Autodesk Inventor part; units mm, degrees
ref_plane "YZ Plane" through (0, 0, 0) normal (1, 0, 0) x (0, 1, 0)
ref_plane "XZ Plane" through (0, 0, 0) normal (0, 1, 0) x (-1, 0, 0)
ref_plane "XY Plane" through (0, 0, 0) normal (0, 0, 1) x (1, 0, 0)
sketch "Sketch1" plane through (0, 0, 0) normal (0, 0, 1) x (1, 0, 0)
  line L0 (15.75, -68) -> (15.75, -43)
  line L1 (15.75, -43) -> (18.75, -43)
  line L2 (18.75, -43) -> (18.75, -68)
  line L3 (43.75, -58) -> (43.75, 0)
  arc A0 (33.75, -68) -> (43.75, -58) centre (33.75, -58) ccw
  circle A1 centre (33.75, -58) radius 5
  line L4 (13.75, 0) -> (13.75, 3)
  line L5 (13.75, 3) -> (3.75, 3)
  line L6 (3.75, 3) -> (3.75, 0)
  line L7 (28.75, 0) -> (28.75, 3)
  line L8 (28.75, 3) -> (38.75, 3)
  line L9 (38.75, 3) -> (38.75, 0)
  line L10 (43.75, 0) -> (38.75, 0)
  line L11 (28.75, 0) -> (13.75, 0)
  line L12 (3.75, 0) -> (0, 0)
  line L13 (0, 0) -> (0, -21.8755)
  line L14 (5.75, -68) -> (0.0154, -22.1236)
  arc A2 (0, -21.8755) -> (0.0154, -22.1236) centre (2, -21.8755) ccw
  line L15 (33.75, -68) -> (18.75, -68)
  line L16 (15.75, -68) -> (5.75, -68)
  line L17 (26.8402, -47) -> (33.75, -47)
  line L18 (38.75, -42) -> (38.75, -10)
  line L19 (22.368, -44.2361) -> (19.2779, -38.0557)
  line L20 (33.75, -5) -> (23.75, -5)
  line L21 (18.75, -10) -> (18.75, -35.8197)
  arc A3 (23.75, -5) -> (18.75, -10) centre (23.75, -10) ccw
  arc A4 (38.75, -10) -> (33.75, -5) centre (33.75, -10) ccw
  arc A5 (33.75, -47) -> (38.75, -42) centre (33.75, -42) ccw
  arc A6 (22.368, -44.2361) -> (26.8402, -47) centre (26.8402, -42) ccw
  arc A7 (18.75, -35.8197) -> (19.2779, -38.0557) centre (23.75, -35.8197) ccw
  point P0 (43.75, -69.5)
  point P1 (0, -22)
  point P2 (23.75, -47)
  point P3 (18.75, -37)
  dimension "d7" = 10
  dimension "d12" = 10
  dimension "d17" = 10
  dimension "d18" = 3
  dimension "d20" = 10
  dimension "d21" = 3
  dimension "d22" = 5
  dimension "d23" = 15
  dimension "d24" = 3
  dimension "d25" = 3
  dimension "d42" = 3
  dimension "d46" = 3.75
  dimension "d47" = 22
  dimension "d49" = 2
  dimension "d54" = 10
  dimension "d55" = 15
  dimension "d57" = 68
  dimension "d58" = 15.75
  dimension "d59" = 25
  dimension "d61" = 5
  dimension "d65" = 5
  dimension "d66" = 10
  dimension "d67" = 5
  dimension "d68" = 5
extrude "Extrusion2" add sketch "Sketch1" along normal blind 3
properties part number "OpenROV 2_3 Dev Handle1"
Read the model definition and answer for the solid it produces. Units are mm, in the model's axes. A direction names the side the tool comes from. Coordinates: 2 decimals unless noted, no trailing zeros. Loops run counter-clockwise (first coordinate to the right, second up) from the corner with the lowest first, then second, coordinate; pieces in that order, holes last. Notation, with made-up numbers: (42, -16.5) -> (85, -16.5) arc R7 cw to (85, -8.5) -> close; hole circle Ø11 at (4.5, 42.5). An arc over 180 degrees is marked (long way). Write item = value, one per line. Start each with the question number.
1) The part is cut by section A-A, the plane z = 1.05. State how many separate pieces and enclosed holes the cut face has, plus the area to 3 significant figures.
2) Given P1, Ø1.5, axis at x = 23, z = 2, coming from the +Y side; P2, Ø1.5, axis at y = 2, z = 2, coming from the +X side; P3, Ø0.9, axis at y = 2, z = 1, coming from the -X side, each flat-ended and moving along its own axis, determine where each tip first touches the part or whether it passes through.
3) The part is cut by section C-C, the plane x = 36. Determine the outline of the cut face in (y, z).
4) For faces 1 (the face through (3.75, 2, 1)), 2 (the face through (18.888, -36.984, 1.479)), 3 (the face through (28.75, 1, 1)), determine the directions among +Z, -Z, +X, -X, +Y, -Y from which every point of the face is accessible in a straight line to the end or side of a thin tool.
5) Find the intervals of material crossed by L1, parallel to Y at x = 33.75, z = 1.8; L2, parallel to X at y = -10, z = 1.85; L3, parallel to Y at x = 33, z = 2, in increasing order. Write a range as from..to.
6) The part is cut by section D-D, the plane y = -62. Determine the outline of the cut face in (x, z), plus the area to 3 significant figures.
7) The part is cut by section B-B, the plane y = -30. Determine the outline of the cut face in (x, z).
8) The mould has two halves that part along Y. Classify faces 4 (the face through (17, -32, 0)), 5 (the face through (17, -43, 1)), 6 (the face through (24.24, -46.27, 1.48)): pulls with the +Y half, pulls with the -Y half, needs draft (parallel to the pull), parting line crosses it, or undercut.
Result:
q1.separate_pieces = 1
q1.enclosed_holes = 2
q1.area = 1,930 mm²
q2.P1 = 0
q2.P2 = 38.75
q2.P3 = 3.75
q3.outline = (-67.74, 0) -> (-62.47, 0) -> (-62.47, 3) -> (-67.74, 3) -> close; (-53.53, 0) -> (-46.47, 0) -> (-46.47, 3) -> (-53.53, 3) -> close; (-5.53, 0) -> (3, 0) -> (3, 3) -> (-5.53, 3) -> close
q4.face_1 = +Z, -Z, -X, +Y
q4.face_2 = +Z, -Z
q4.face_3 = +Z, -Z, +Y
q5.L1 = -68..-63, -53..-47, -5..3
q5.L2 = 0..18.75, 38.75..43.75
q5.L3 = -68..-62.94, -53.06..-47, -5..3
q6.outline = (5, 0) -> (15.75, 0) -> (15.75, 3) -> (5, 3) -> close; (18.75, 0) -> (30.75, 0) -> (30.75, 3) -> (18.75, 3) -> close; (36.75, 0) -> (42.92, 0) -> (42.92, 3) -> (36.75, 3) -> close
q6.area = 86.7 mm²
q7.outline = (1, 0) -> (18.75, 0) -> (18.75, 3) -> (1, 3) -> close; (38.75, 0) -> (43.75, 0) -> (43.75, 3) -> (38.75, 3) -> close
q8.face_4 = needs draft
q8.face_5 = pulls with the -Y half
q8.face_6 = undercut
